Drawing for the job (mm, zero at the part's lowest x, y, z). A direction names the side the tool comes from. Give positions to 0.01 mm unless a question says otherwise; leave off trailing zeros. Order: outer loops, then holes, each group sorted by start corner. A loop starts at its lowest first (then second) coordinate and runs counter-clockwise, first axis right, second up. Notation, with made-up numbers: M 64,84.25 L 119,84.25 A15 ccw 119,101.25 Z; hole C -22,37 d4. An arc over 180 degrees is marked long. One line per item, written item: value.
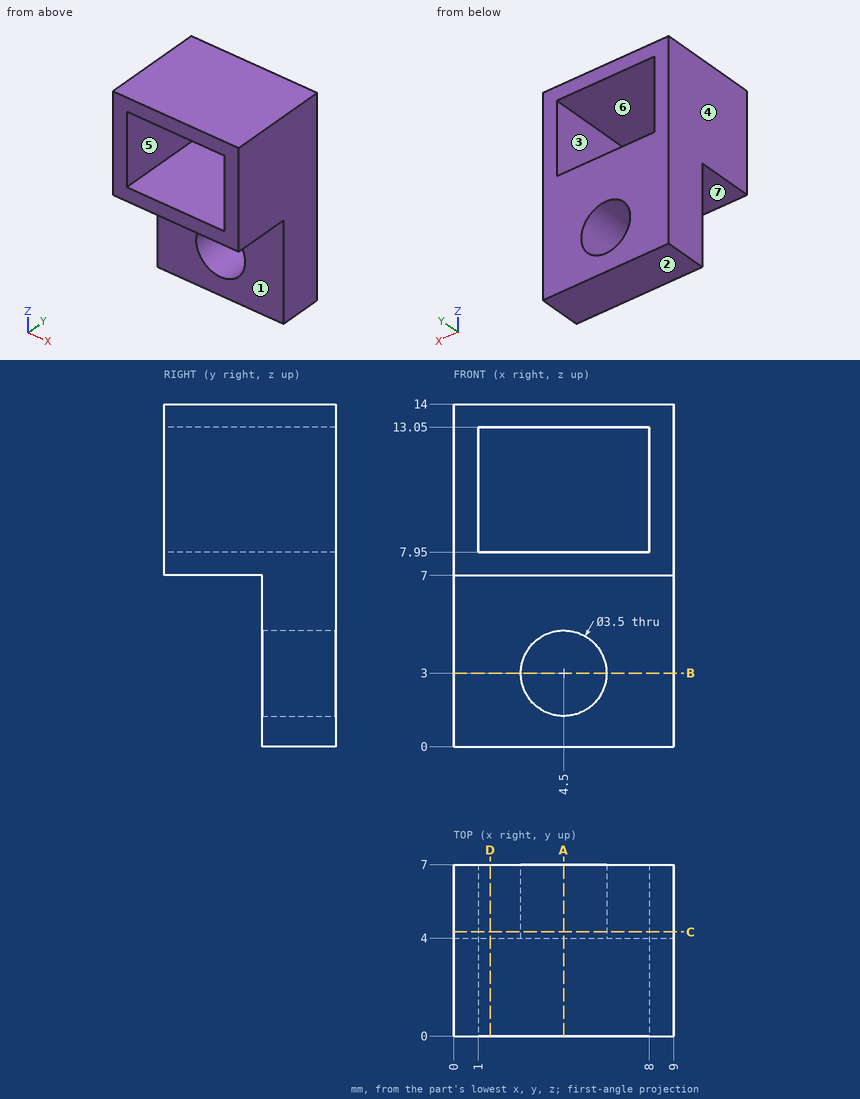
1) Saw through at C-C, the plane y = 4.25. Write the cut outline in (x, z).
Check values:
outline: M 0,0 L 9,0 L 9,14 L 0,14 Z; hole M 1,7.95 L 8,7.95 L 8,13.05 L 1,13.05 Z; hole C 4.5,3 d3.5
2) Saw through at D-D, the plane x = 1.5. Write the cut outline in (y, z).
Check values:
outline: M 0,7 L 4,7 L 4,0 L 7,0 L 7,7.95 L 0,7.95 Z; M 0,13.05 L 7,13.05 L 7,14 L 0,14 Z
3) Mould opens along X. For the marked faces 4, 5, 6 and 7 say: released by +X, released by -X, zero draft, split by the parting line, or undercut.
Check values:
face 4: released by -X
face 5: undercut
face 6: undercut
face 7: zero draft
4) Drill centre lines: probe 1 along Z at (x, y) = (4.5, 5.8); probe 2 along X at (y, z) = (5, 3); probe 3 along Z at (x, y) = (1.5, 5.5). Where is each one in solid material? Low to high. Write a range as from..to.
Check values:
probe 1: 0..1.25, 4.75..7.95, 13.05..14
probe 2: 0..2.75, 6.25..9
probe 3: 0..7.95, 13.05..14
5) Saw through at B-B, the plane z = 3. Write the cut outline in (x, y), then the cut area to 3 significant figures.
Check values:
outline: M 0,4 L 2.75,4 L 2.75,7 L 0,7 Z; M 6.25,4 L 9,4 L 9,7 L 6.25,7 Z
area: 16.5 mm^2
6) Saw through at A-A, the plane x = 4.5. Write the cut outline in (y, z), then the cut area to 3 significant figures.
Check values:
outline: M 0,7 L 4,7 L 4,4.75 L 7,4.75 L 7,7.95 L 0,7.95 Z; M 0,13.05 L 7,13.05 L 7,14 L 0,14 Z; M 4,0 L 7,0 L 7,1.25 L 4,1.25 Z
area: 23.8 mm^2
7) Tool access for the marked faces 1, 2 and 3: list every direction of +Z, -Z, +X, -X, +Y, -Y with a clear straight run to the whole face (end or side of a thin tool).
Check values:
face 1: -Z, +X, -X, -Y
face 2: -Z, +X, -X, +Y, -Y
face 3: +Y, -Y
8) Pin check, flat tips, straight feed: pin 1 (1.2 mm diameter, centred on x = 4.5, y = 2.5, fed in from -Z); pin 2 (2.5 mm diameter, centred on y = 2.5, z = 10.5, fed in from -X). Stop position of each tip, or through.
Check values:
pin 1: z = 7
pin 2: x = 0
